Study the drawing (mm; zero at the part's minimum x, y, z) and answer. A direction names the side the tool comes from. Coordinates: 2 decimals unless noted, no trailing zeros. Order: outer loops, then holes, each group sorted by start corner. A loop starts at its lowest first (then second) coordinate and runs counter-clockwise, first axis right, second up.
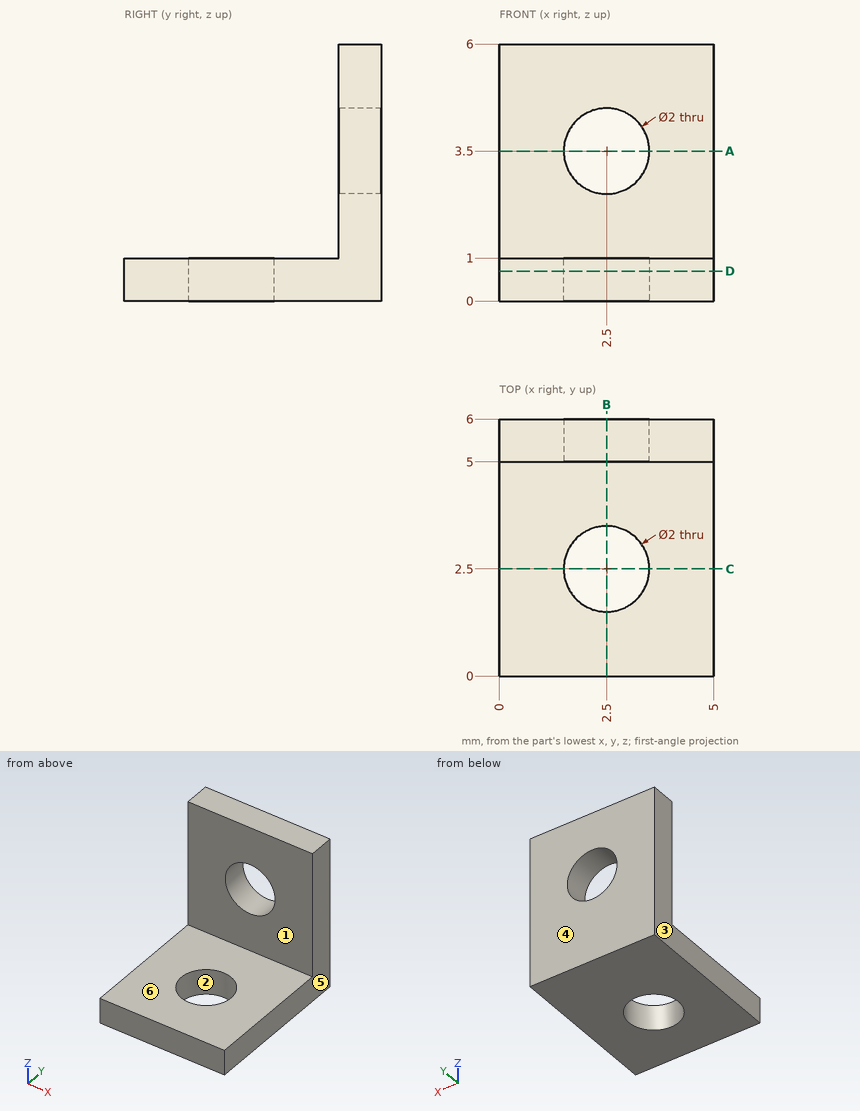
(1) Find section D-D (z = 0.7). Write down the section's boundary in (x, y).
(2) Find section A-A (z = 3.5). Write down the section's boundary in (x, y), and give its area (3 significant figures).
(3) Find section C-C (y = 2.5). Write down the section's boundary in (x, z).
(4) Each of these flat-tipped pins is pushed along its axis until it touches: pin 1 Ø2.5 at (x, y) = (3, 3.5) entering from +Z; pin 2 Ø1 at (x, z) = (3.5, 5) entering from -Y; pin 3 Ø1.6 at (x, z) = (2.5, 3.5) entering from +Y. Where does it stop, or does it pass through?
(5) The mould has two halves that part along Y. Classify the marked faces 1, 2, 3 and 4: released by +Y, released by -Y, zero draft, split by the parting line, or undercut.
(6) Consider line 1 (Z direction, x = 2.5, y = 5.3); line 2 (Y direction, x = 2.5, z = 0.4); line 3 (Y direction, x = 2.7, z = 4.65). Determine where each line is inside the solid, lowest interval first.
(7) For the marked faces 5 and 6, determine the directions among +Z, -Z, +X, -X, +Y, -Y from which every point of the face is accessible in a straight line to the end or side of a thin tool.
(8) Find section B-B (x = 2.5). Write down the section's boundary in (y, z), and give its area (3 significant figures).
Findings below:
1. outline: (0, 0) - (5, 0) - (5, 6) - (0, 6) - close; hole circle Ø2 at (2.5, 2.5)
2. outline: (0, 5) - (1.5, 5) - (1.5, 6) - (0, 6) - close; (3.5, 5) - (5, 5) - (5, 6) - (3.5, 6) - close
2. area: 3.00 mm2
3. outline: (0, 0) - (1.5, 0) - (1.5, 1) - (0, 1) - close; (3.5, 0) - (5, 0) - (5, 1) - (3.5, 1) - close
4. pin 1: stops at z = 1
4. pin 2: stops at y = 5
4. pin 3: passes through
5. face 1: released by -Y
5. face 2: undercut
5. face 3: zero draft
5. face 4: released by +Y
6. line 1: z = 0 to 2.5, 4.5 to 6
6. line 2: y = 0 to 1.5, 3.5 to 6
6. line 3: y = 5 to 6
7. face 5: +Z, -Z, +X, +Y, -Y
7. face 6: +Z, +X, -X, -Y
8. outline: (0, 0) - (1.5, 0) - (1.5, 1) - (0, 1) - close; (3.5, 0) - (6, 0) - (6, 2.5) - (5, 2.5) - (5, 1) - (3.5, 1) - close; (5, 4.5) - (6, 4.5) - (6, 6) - (5, 6) - close
8. area: 7.00 mm2
